Solid Edge part; units mm, degrees
sketch "Sketch1" plane through (0, 0, 0) normal (0, 0, 1) x (1, 0, 0)
  circle A0 centre (0, 0) radius 3.5
extrude "Protrusion1" add sketch "Sketch1" along normal blind 4
sketch "Sketch2" plane through (0, 0, 4) normal (0, 0, 1) x (0, 1, 0)
  line L0 (0, 1.7321) -> (1.5, 0.866)
  line L1 (1.5, 0.866) -> (1.5, -0.866)
  line L2 (1.5, -0.866) -> (0, -1.7321)
  line L3 (0, -1.7321) -> (-1.5, -0.866)
  line L4 (-1.5, -0.866) -> (-1.5, 0.866)
  line L5 (-1.5, 0.866) -> (0, 1.7321)
extrude "Cutout1" cut sketch "Sketch2" against normal blind 2
fillet "Round1" radius 0.4 1 edges at (-3.5, 0, 4)
sketch "Sketch3" plane through (0, 0, 0) normal (1, 0, 0) x (0, 1, 0)
  line L0 (-1.5705, -10) -> (0, -10)
  line L1 (-2, -9.5705) -> (-1.5705, -10)
  line L2 (-2, -2.1) -> (-2, -9.5705)
  line L3 (-1.5705, -2.1) -> (-2, -2.1)
  line L4 (-1.5705, -2.09) -> (-1.5705, -2.1)
  line L5 (-2, -2.09) -> (-1.5705, -2.09)
  line L6 (-2, -0.2) -> (-2, -2.09)
  arc A0 (-2, -0.2) -> (-2.2, 0) centre (-2.2, -0.2) ccw
revolve "RevolvedProtrusion1" add sketch "Sketch3" angle 360 about axis through (0, 0, -60.325) along (0, 0, 1) material side at (0, -0.7853, -9.95)
cosmetic_thread "Thread1"
sketch "Sketch4" plane through (0, 0, 0) normal (0, -1, 0) x (1, 0, 0)
  line L0 (-1.72, 4) -> (0, 3.007)
revolve "RevolvedCutout1" cut sketch "Sketch4" angle 360 about axis through (0, 0, 57.15) along (0, 0, -1) material side at (-0.835, 0, 3.5468)
properties material "Stahl"
For this review, take the finished solid that the model builds, in its own axes (mm). A direction names the side the tool comes from. Give positions to 0.01 mm unless a question says otherwise; leave off trailing zeros. Loops run counter-clockwise (first coordinate to the right, second up) from the corner with the lowest first, then second, coordinate; pieces in that order, holes last. Notation, with made-up numbers: (63, 41.5) - (112, 41.5) arc R19 ccw to (112, 53.5) - close; hole circle Ø7 at (36, 32). An arc over 180 degrees is marked (long way). Write each question's results on one line, items separated by ' | '.
(1) Draft analysis for pull direction Y (two halves, no side actions). For faces 1 (the flat face through (0, 0, 2)), 2 (the flat face through (1.33, -1.33, 4)), 3 (the cylindrical face through (3.233, 1.341, 1.775)), state which applies: +Y half, -Y half, draft (parallel to the pull), parting line (faces both ways), or undercut.
Conclusion:
face 1: undercut | face 2: draft | face 3: parting line
(2) For line 1 along Z through (x, y) = (2.25, 2); line 2 along Y through (x, z) = (1.5, 2.5); line 3 along Z through (x, y) = (0, -1), list the stretches that pass through material, from the lowest coordinate up.
Conclusion:
line 1: 0 to 4 | line 2: -3.16 to -0.4, 0.4 to 3.16 | line 3: -10 to 2
(3) Take a section at C-C (z = -9). Give the boundary of the cut face in (x, y).
Conclusion:
outline: circle Ø4 at (0, 0)
(4) For faces 4 (the flat face through (0, 0, -10)), 5 (the flat face through (0, 1.5, 3)), 6 (the flat face through (-2, -2, 0)), list the 3-axis set-ups (+Z, -Z, +X, -X, +Y, -Y) from which the entire face can be reached by the end or side of a thin tool; tool diameter is ignored.
Conclusion:
face 4: -Z, +X, -X, +Y, -Y | face 5: +Z | face 6: -Z
(5) Take a section at B-B (z = 1.25). Give the boundary of the cut face in (x, y), then the cut area to 3 significant figures.
Conclusion:
outline: circle Ø7 at (0, 0) | area: 38.5 mm^2
(6) For pin 1 Ø0.9 at (x, y) = (-0.5, 0) entering from +Z; pin 2 Ø0.5 at (x, z) = (0.5, 2.5) entering from -Y; pin 3 Ø4 at (y, z) = (-2.5, 2) entering from -X, all flat-tipped, find the tip position at first contact; note any pin that passes through.
Conclusion:
pin 1: z = 2 | pin 2: y = -3.49 | pin 3: x = -3.46
